Read the model definition and answer for the solid it produces. Units are mm, in the model's axes. Face numbers are marked on the shaded views. A direction names the side the tool comes from. Give positions to 0.01 mm unless a question says otherwise; leave off trailing zeros. Order: outer loops, then holes, each group sorted by start corner. A loop starts at its lowest first (then second) coordinate and runs counter-clockwise, first axis right, second up.
Item 1: A cutting plane is placed at A-A (y = 37.5). Write down the section's boundary in (x, z).
Item 2: Given pin 1 Ø2 at (x, z) = (-245.5, 1) entering from +Y; pin 2 Ø5 at (x, y) = (221.5, 18.5) entering from +Z; pin 3 Ø7.5 at (x, z) = (-121, 9) entering from +Y, each flat-ended and moving along its own axis, determine where each tip first touches the part or whether it passes through.
Item 3: Which of the six approach directions +Z, -Z, +X, -X, +Y, -Y give full straight-line access (tool end or side, diameter ignored) to the marked faces 1 and 2?
Item 4: A cutting plane is placed at B-B (x = 157). Write down the section's boundary in (y, z).
Item 5: Find the intervals of material crossed by line 1 along X through (y, z) = (47.5, 1); line 2 along Z through (x, y) = (435, 49.5); line 3 along Y through (x, z) = (-233, 12), in increasing order.
Item 6: A cutting plane is placed at C-C (z = 14.25). Write down the section's boundary in (x, y).
Autodesk Inventor part; units mm, degrees
ref_plane "YZ Plane" through (0, 0, 0) normal (1, 0, 0) x (0, 1, 0)
ref_plane "XZ Plane" through (0, 0, 0) normal (0, 1, 0) x (-1, 0, 0)
ref_plane "XY Plane" through (0, 0, 0) normal (0, 0, 1) x (1, 0, 0)
sketch "Sketch1" plane through (0, 0, 0) normal (0, 0, 1) x (1, 0, 0)
  line L0 (-490, 72) -> (490, 72)
  line L1 (490, 72) -> (490, 0)
  line L2 (490, 0) -> (-490, 0)
  line L3 (-490, 0) -> (-490, 72)
  point P0 (0, 0)
  point P1 (0, 0)
  dimension "d0" = 980
  dimension "d1" = 72
extrude "Plate1" add sketch "Sketch1" along normal blind 2
sketch "Sketch2" plane through (490, -2, 0) normal (0, 1, 0) x (-1, 0, 0)
  line L0 (980, 0) -> (0, 0)
  line L1 (0, 0) -> (0, 20)
  line L2 (0, 20) -> (980, 20)
  line L3 (980, 20) -> (980, 0)
edge flange "Flange1" height 20 angle 90 thickness 2 bend radius 2.75 thickness toward (0, 1, 0) relief round relief width 2 relief depth 1 edges at (0, 0, 2) wall of the first edge with corners at (-490, -2, 0) (490, -2, 0) (490, -2, 20) (-490, -2, 20)
bend "Bend1"
corner "Corner1"
sketch "Sketch5" plane through (0, 0, 0) normal (0, 0, -1) x (-1, 0, 0)
  line L0 (490, 72) -> (-490, 72)
  line L1 (490, -2) -> (-490, -2)
  circle A0 centre (0, 72) radius 17.5
  line L2 (243.4, 72) -> (246.6, 72)
  line L3 (246.6, 72) -> (246.6, 26)
  line L4 (246.6, 26) -> (243.4, 26)
  line L5 (243.4, 26) -> (243.4, 72)
  line L6 (-243.4, 72) -> (-246.6, 72)
  line L7 (-246.6, 72) -> (-246.6, 26)
  line L8 (-246.6, 26) -> (-243.4, 26)
  line L9 (-243.4, 26) -> (-243.4, 72)
  line L10 (0, 72) -> (0, -2) construction
  line L11 (-490, -2) -> (-490, 72)
  line L12 (490, -2) -> (490, 72)
  circle A1 centre (-490, 72) radius 17.5
  circle A2 centre (490, 72) radius 17.5
  point P0 (0, 0)
  point P1 (245, 26)
  point P2 (-245, 26)
  point P3 (246.6, 72)
  point P4 (-17.5, 72)
  point P5 (17.5, 72)
  point P6 (-246.6, 72)
  point P7 (472.5, 72)
  point P8 (490, 54.5)
  point P9 (-490, 54.5)
  point P10 (-472.5, 72)
  dimension "d45" = 35
  dimension "d48" = 3.2
  dimension "d49" = 490
  dimension "d51" = 28
  dimension "d52" = 46
extrude "Extrusion1" cut sketch "Sketch5" against normal through all contours L3 L4 L5 L0 | L0 L12 A2 | L9 L8 L7 L0 | L11 L0 A1 picked at (478.4796, 70.702) picked at (-478.4796, 70.702)
sketch "Sketch9" plane through (0, 0, 2) normal (0, 0, 1) x (1, 0, 0)
  line L0 (467.0539, 27.7998) -> (467.0539, 15.7998) construction
  line L1 (467.0539, 15.7998) -> (267.0539, 15.7998) construction
  line L2 (267.0539, 15.7998) -> (267.0539, 27.7998) construction
  line L3 (267.0539, 27.7998) -> (467.0539, 27.7998) construction
  line L4 (-490, 72) -> (490, 72)
  point P0 (0, 0)
  point P1 (1.05, 68)
  point P2 (490, 72)
  point P3 (-490, 72)
  dimension "d40" = 200
  dimension "d41" = 12
mark "Mark2"
equation "\"d2\" = Thickness"
equation "\"d3\" = BendReliefWidth"
equation "\"d4\" = BendReliefDepth"
equation "\"d5\" = MinimumRemnant"
equation "\"d6\" = TransitionRadius"
equation "\"d9\" = BendRadius"
equation "\"d10\" = CornerReliefSize"
equation "\"d11\" = GapSize"
equation "\"d12\" = JacobiRadiusSize"
equation "\"BendReliefWidth\" = Thickness"
equation "\"BendReliefDepth\" = 0.5 * Thickness"
equation "\"CornerReliefSize\" = 4 * Thickness"
equation "\"MinimumRemnant\" = 2 * Thickness"
equation "\"TransitionRadius\" = BendRadius"
equation "\"JacobiRadiusSize\" = BendRadius"
equation "\"GapSize\" = Thickness"
properties part number "MSC 344 stringer BOARD  ####" material "Stainless Steel"
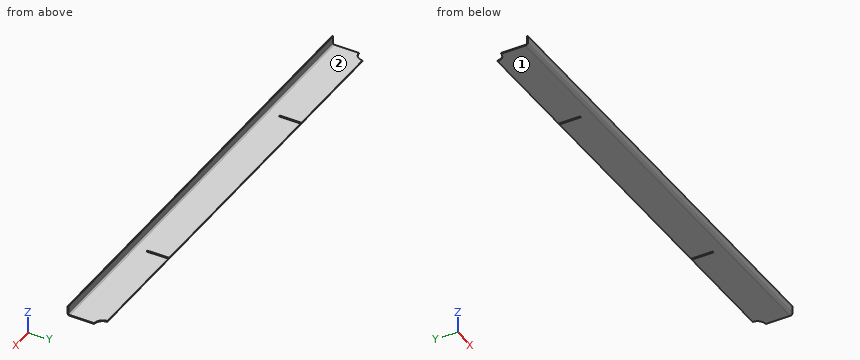
Response values:
1. outline: (-490, 0) - (-246.6, 0) - (-246.6, 2) - (-490, 2) - close; (-243.4, 0) - (243.4, 0) - (243.4, 2) - (-243.4, 2) - close; (246.6, 0) - (490, 0) - (490, 2) - (246.6, 2) - close
2. pin 1: stops at y = 26
2. pin 2: stops at z = 2
2. pin 3: stops at y = 0
3. face 1: -Z, +X, -X, +Y, -Y
3. face 2: +Z, +X, -X, +Y
4. outline: (-2, 4.75) arc R4.75 ccw to (2.75, 0) - (72, 0) - (72, 2) - (2.75, 2) arc R2.75 cw to (0, 4.75) - (0, 20) - (-2, 20) - close
5. line 1: x = -490 to -246.6, -243.4 to 243.4, 246.6 to 490
5. line 2: z = 0 to 2
5. line 3: y = -2 to 0
6. outline: (-490, -2) - (490, -2) - (490, 0) - (-490, 0) - close
